```python
from build123d import *

# Parameters (mm, degrees)
RESSALTO_EXTRUS_O1_DEPTH = 3


with BuildPart() as part:
    # Esboço1 → Ressalto-extrusão1 (new body)
    with BuildSketch(Plane.XY):
        with BuildLine():
            Line((3, 0), (7, 0))
            Line((7, 0), (7, 3))
            Line((7, 3), (7, 4.5))
            Line((7, 4.5), (10, 4.5))
            Line((10, 4.5), (10, 3))
            Line((10, 3), (10, 0))
            Line((10, 0), (10, -0.015366586))
            ThreePointArc((10, -0.015366586), (9.570424226, -1.990324177), (8.359319479, -3.608415065))
            ThreePointArc((8.359319479, -3.608415065), (7.72499373, -4.455903043), (7.5, -5.490302797))
            Line((7.5, -5.490302797), (7.5, -6.25))
            Line((7.5, -6.25), (7.5, -12.5))
            Line((7.5, -12.5), (7.5, -15))
            ThreePointArc((7.5, -15), (9.550252532, -19.949747468), (14.5, -22))
            Line((14.5, -22), (15, -22))
            Line((15, -22), (15, -25))
            Line((15, -25), (-5, -25))
            Line((-5, -25), (-5, -22))
            Line((-5, -22), (-4.5, -22))
            ThreePointArc((-4.5, -22), (0.449747468, -19.949747468), (2.5, -15))
            Line((2.5, -15), (2.5, -12.5))
            Line((2.5, -12.5), (2.5, -6.25))
            Line((2.5, -6.25), (2.5, -5.490302797))
            ThreePointArc((2.5, -5.490302797), (2.270627847, -4.446367624), (1.62476455, -3.594738109))
            ThreePointArc((1.62476455, -3.594738109), (0.425800558, -2.013795009), (0, -0.075860639))
            Line((0, -0.075860639), (0, 0))
            Line((0, 0), (0, 3))
            Line((0, 3), (0, 4.5))
            Line((0, 4.5), (3, 4.5))
            Line((3, 4.5), (3, 3))
            Line((3, 3), (3, 0))
        make_face()
    extrude(amount=RESSALTO_EXTRUS_O1_DEPTH)


solid = part.part
```
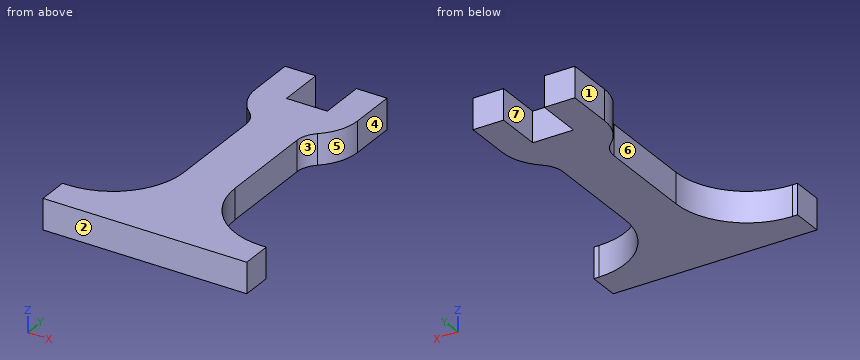
The model under review builds one solid part; all positions refer to its coordinate system, in mm. Face numbers are marked on the shaded views. A direction names the side the tool comes from. Coordinates: 2 decimals unless noted, no trailing zeros. Loops run counter-clockwise (first coordinate to the right, second up) from the corner with the lowest first, then second, coordinate; pieces in that order, holes last. Notation, with made-up numbers: (58.25, 46.25) -> (110.25, 46.25) arc R31 cw to (110.25, 81.25) -> close; hole circle Ø3 at (13, -24). An arc over 180 degrees is marked (long way). Answer as CSV lines item,"result".
Item 1: For L1, parallel to X at y = 3.75, z = 1.25; L2, parallel to X at y = -13.5, z = 0.65; L3, parallel to Y at x = 6, z = 2.8, list the stretches that pass through material, from the lowest coordinate up.
Results below:
L1,"x = 0 to 3, 7 to 10"
L2,"x = 2.5 to 7.5"
L3,"y = -25 to 0"
Item 2: Take a section at C-C, the plane z = 2.45. State the section outline as (x, y) points, and give its area (3 significant figures).
Results below:
outline,"(-5, -25) -> (15, -25) -> (15, -22) -> (14.5, -22) arc R7 cw to (7.5, -15) -> (7.5, -5.49) arc R2.49 cw to (8.36, -3.61) arc R4.75 ccw to (10, -0.02) -> (10, 4.5) -> (7, 4.5) -> (7, 0) -> (3, 0) -> (3, 4.5) -> (0, 4.5) -> (0, -0.08) arc R4.62 ccw to (1.62, -3.59) arc R2.49 cw to (2.5, -5.49) -> (2.5, -15) arc R7 cw to (-4.5, -22) -> (-5, -22) -> close"
area,"233 mm2"
Item 3: Take a section at D-D, the plane x = 6.25. State the section outline as (y, z) points, and give its area (3 significant figures).
Results below:
outline,"(-25, 0) -> (0, 0) -> (0, 3) -> (-25, 3) -> close"
area,"75.0 mm2"
Item 4: Draft analysis for pull direction Y (two halves, no side actions). For the marked faces 1, 2 and 3, state which applies: +Y half, -Y half, draft (parallel to the pull), parting line (faces both ways), or undercut.
Results below:
face 1,"draft"
face 2,"-Y half"
face 3,"undercut"
Item 5: Take a section at A-A, the plane y = 0.75. State the section outline as (x, z) points, and give its area (3 significant figures).
Results below:
outline,"(0, 0) -> (3, 0) -> (3, 3) -> (0, 3) -> close; (7, 0) -> (10, 0) -> (10, 3) -> (7, 3) -> close"
area,"18.0 mm2"
Item 6: Take a section at B-B, the plane x = 2. State the section outline as (y, z) points.
Results below:
outline,"(-25, 0) -> (-17.6, 0) -> (-17.6, 3) -> (-25, 3) -> close; (-3.99, 0) -> (4.5, 0) -> (4.5, 3) -> (-3.99, 3) -> close"
Item 7: Machinability: for the marked faces 4, 5, 6 and 7, which of the approach directions +Z, -Z, +X, -X, +Y, -Y give a long, thin tool a straight path to every point of the face, cutting with its end or side? Answer none if there is none.
Results below:
face 4,"+Z, -Z, +X, +Y"
face 5,"+Z, -Z, +X"
face 6,"+Z, -Z, -X"
face 7,"+Z, -Z, +Y"
Item 8: Insertion check: pin 1 (1.5 mm diameter, centred on y = 1.5, z = 2, fed in from +X); pin 2 (1.5 mm diameter, centred on y = 2.5, z = 1, fed in from -X); pin 3 (0.9 mm diameter, centred on y = -11, z = 1.5, fed in from -X). Each pin has a flat end and moves straight along its axis. Give the tip position at first contact, or say it passes through.
Results below:
pin 1,"stops at x = 10"
pin 2,"stops at x = 0"
pin 3,"stops at x = 2.5"
